from build123d import *

# Parameters (mm, degrees)
MASTER_SKETCH_R       = 52.451
MASTER_SKETCH_R_2     = 9.525
MASTER_SKETCH_R_3     = 45.974
MASTER_SKETCH_R_4     = 27.4955
MASTER_SKETCH_R_5     = 5.5
BOSS_EXTRUDE2_DEPTH   = 6.096
F_5_0MM_DOWEL_HOLE1_D = 5
CIRPATTERN4_COUNT     = 4
M6_CLEARANCE_HOLE4_D  = 6.6
M8_CLEARANCE_HOLE1_D  = 9
CIRPATTERN3_COUNT     = 18
CUT_EXTRUDE1_DEPTH    = 284.854467488


with BuildPart() as part:
    # Master Sketch → Boss-Extrude2 (new body)
    # profile 1 of 5: a face of its own
    with BuildSketch(Plane(origin=(0, 0, 0), x_dir=(1, 0, 0), z_dir=(0, 1, 0))):
        with BuildLine():
            ThreePointArc((-8.636, 127), (-36.396097826, 84.787887478), (-86.152093601, 93.552952189))
            Line((-86.152093601, 93.552952189), (-6.534964144, 18.470363023))
            ThreePointArc((-6.534964144, 18.470363023), (-3.773598517, 34.145603423), (9.525, 25.4))
            ThreePointArc((9.525, 25.4), (8.799952547, 21.754940307), (6.735192091, 18.664807909))
            Line((6.735192091, 18.664807909), (34.255961574, 46.185577392))
            ThreePointArc((34.255961574, 46.185577392), (59.945142207, 60.02346539), (89.010077776, 57.44457682))
            Line((89.010077776, 57.44457682), (207.987004211, 9.951947906))
            ThreePointArc((207.987004211, 9.951947906), (204.851852042, 25.601533276), (220.43444462, 22.148779315))
            Line((220.43444462, 22.148779315), (189.133864847, 105.44289655))
            ThreePointArc((189.133864847, 105.44289655), (188.207777178, 115.4635324), (192.51641215, 124.557840832))
            Line((192.51641215, 124.557840832), (212.800120602, 148.168522003))
            ThreePointArc((212.800120602, 148.168522003), (196.940842995, 150.353698677), (205.472725722, 163.899866417))
            Line((205.472725722, 163.899866417), (169.599038165, 163.514054819))
            ThreePointArc((169.599038165, 163.514054819), (163.800537316, 164.352688386), (158.531122559, 166.913779261))
            ThreePointArc((158.531122559, 166.913779261), (141.706259737, 175.147152322), (123.19, 177.9778))
            Line((123.19, 177.9778), (-54.61, 172.974))
            ThreePointArc((-54.61, 172.974), (-22.101472842, 159.508527158), (-8.636, 127))
        make_face()
        with Locations(Location((123.19, 116.0018, 0), (0, 0, 90))):
            Circle(MASTER_SKETCH_R, mode=Mode.SUBTRACT)
    # profile 2 of 5: a face of its own
    with BuildSketch(Plane(origin=(0, 0, 0), x_dir=(1, 0, 0), z_dir=(0, 1, 0))):
        with Locations((0, 25.4)):
            Circle(MASTER_SKETCH_R_2)
    # profile 3 of 5: a face of its own
    with BuildSketch(Plane(origin=(0, 0, 0), x_dir=(1, 0, 0), z_dir=(0, 1, 0))):
        with Locations((211.518208908, 18.79820239)):
            Circle(MASTER_SKETCH_R_2)
    # profile 4 of 5: a face of its own
    with BuildSketch(Plane(origin=(0, 0, 0), x_dir=(1, 0, 0), z_dir=(0, 1, 0))):
        with Locations((205.575158542, 154.375417219)):
            Circle(MASTER_SKETCH_R_2)
    # profile 5 of 5: a face of its own
    with BuildSketch(Plane(origin=(0, 0, 0), x_dir=(1, 0, 0), z_dir=(0, 1, 0))):
        with Locations((-54.61, 127)):
            Circle(MASTER_SKETCH_R_3)
        with Locations(Location((-54.61, 127, 0), (0, 0, 90))):
            Circle(MASTER_SKETCH_R_4, mode=Mode.SUBTRACT)
        with Locations(Location((-41.27121441, 90.351987789, 0), (0, 0, 90))):
            Circle(MASTER_SKETCH_R_5, mode=Mode.SUBTRACT)
        with Locations(Location((-67.94878559, 90.351987789, 0), (0, 0, 90))):
            Circle(MASTER_SKETCH_R_5, mode=Mode.SUBTRACT)
    extrude(amount=BOSS_EXTRUDE2_DEPTH)

    # Ø5.0mm Dowel Hole1 (through all)
    with Locations(Plane(origin=(0, 6.096, 0), x_dir=(1, 0, 0), z_dir=(0, 1, 0))):
        with Locations((123.19, 173.14676824)):
            f_5_0mm_dowel_hole1 = Hole(F_5_0MM_DOWEL_HOLE1_D / 2)

    # CirPattern4: Ø5.0mm Dowel Hole1 ×4 about axis
    cirpattern4_axis = Axis((123.19, 0, -116.0018), (0, 1, 0))
    for i in range(1, CIRPATTERN4_COUNT):
        add(f_5_0mm_dowel_hole1.rotate(cirpattern4_axis, i * 360 / CIRPATTERN4_COUNT), mode=Mode.SUBTRACT)

    # M6 Clearance Hole4 (through all)
    with Locations(Plane(origin=(0, 6.096, 0), x_dir=(1, 0, 0), z_dir=(0, 1, 0))):
        with Locations((205.575158542, 154.375417219), (211.518208908, 18.79820239), (0, 25.4)):
            Hole(M6_CLEARANCE_HOLE4_D / 2)

    # M8 Clearance Hole1 (through all)
    with Locations(Plane(origin=(0, 6.096, 0), x_dir=(1, 0, 0), z_dir=(0, 1, 0))):
        with Locations((-54.61, 166)):
            m8_clearance_hole1 = Hole(M8_CLEARANCE_HOLE1_D / 2)

    # CirPattern3: M8 Clearance Hole1 ×18 about axis, 10 skipped
    cirpattern3_axis = Axis((-54.61, 6.096, -127), (0, -1, 0))
    add([m8_clearance_hole1.rotate(cirpattern3_axis, i * 360 / CIRPATTERN3_COUNT) for i in range(1, CIRPATTERN3_COUNT) if i not in (1, 3, 5, 7, 8, 10, 11, 13, 15, 17)], mode=Mode.SUBTRACT)

    # Topology 1 → Cut-Extrude1 (cut, through all)
    with BuildSketch(Plane(origin=(0, 6.096, 0), x_dir=(1, 0, 0), z_dir=(0, 1, 0))):
        with BuildLine():
            ThreePointArc((67.281456447, 150.672141126), (71.26845327, 156.399210575), (75.839660388, 161.67173688))
            ThreePointArc((75.839660388, 161.67173688), (76.458883843, 165.158331399), (73.46509413, 167.049627827))
            Line((73.46509413, 167.049627827), (-14.700169403, 164.56840541))
            ThreePointArc((-14.700169403, 164.56840541), (-17.514771269, 162.678357132), (-17.018226233, 159.324596677))
            ThreePointArc((-17.018226233, 159.324596677), (-13.365554188, 154.512119056), (-10.325367902, 149.291082638))
            ThreePointArc((-10.325367902, 149.291082638), (-7.908159584, 146.693689239), (-4.474760882, 145.79863512))
            Line((-4.474760882, 145.79863512), (62.063515299, 147.671212322))
            ThreePointArc((62.063515299, 147.671212322), (65.050656221, 148.51412343), (67.281456447, 150.672141126))
        make_face()
        with BuildLine():
            ThreePointArc((68.334394598, 79.68843673), (68.764556906, 73.722595945), (63.886881332, 70.260721182))
            ThreePointArc((63.886881332, 70.260721182), (44.213471784, 64.716380715), (27.520769483, 52.920769483))
            Line((27.520769483, 52.920769483), (11.599172261, 36.999172261))
            ThreePointArc((11.599172261, 36.999172261), (9.657159805, 36.083732416), (7.576574711, 36.613457017))
            ThreePointArc((7.576574711, 36.613457017), (-0.198277171, 38.93169571), (-7.901868408, 36.386654554))
            ThreePointArc((-7.901868408, 36.386654554), (-9.966039712, 35.796197685), (-11.934040176, 36.65434491))
            Line((-11.934040176, 36.65434491), (-13.130428791, 37.782594013))
            ThreePointArc((-13.130428791, 37.782594013), (-16.07794783, 41.990645294), (-17.117143266, 47.022109982))
            Line((-17.117143266, 47.022109982), (-17.117143266, 64.392614711))
            ThreePointArc((-17.117143266, 64.392614711), (-14.042484998, 72.677709553), (-6.307254046, 76.95117678))
            Line((-6.307254046, 76.95117678), (59.587432499, 86.868574701))
            ThreePointArc((59.587432499, 86.868574701), (63.174454879, 86.315869277), (65.811602789, 83.822344916))
            ThreePointArc((65.811602789, 83.822344916), (67.034945598, 81.732168237), (68.334394598, 79.68843673))
        make_face()
        with BuildLine():
            ThreePointArc((206.458947193, 32.26142708), (204.959027962, 25.492155206), (198.160653587, 24.130206141))
            Line((198.160653587, 24.130206141), (145.349760257, 45.211000835))
            ThreePointArc((145.349760257, 45.211000835), (142.353542672, 49.714608993), (145.500239117, 54.114393959))
            ThreePointArc((145.500239117, 54.114393959), (164.91203471, 65.138555749), (179.519499105, 82.019667539))
            ThreePointArc((179.519499105, 82.019667539), (184.033435332, 84.302068881), (188.055524715, 81.234859539))
            Line((188.055524715, 81.234859539), (206.458947193, 32.26142708))
        make_face()
        with BuildLine():
            Line((190.604833072, 136.949630286), (196.435820245, 143.737027147))
            ThreePointArc((196.435820245, 143.737027147), (197.375389236, 150.556102986), (191.550890325, 154.22459009))
            Line((191.550890325, 154.22459009), (182.60327011, 154.128360907))
            ThreePointArc((182.60327011, 154.128360907), (179.873089832, 152.515317466), (179.900424771, 149.344348167))
            ThreePointArc((179.900424771, 149.344348167), (182.824339377, 143.778469401), (185.203579034, 137.958890231))
            ThreePointArc((185.203579034, 137.958890231), (187.613336253, 135.897613045), (190.604833072, 136.949630286))
        make_face()
    extrude(amount=-CUT_EXTRUDE1_DEPTH, mode=Mode.SUBTRACT)


solid = part.part
Verification items for the finished model (mm, model axes). A direction names the side the tool comes from. Coordinates: 2 decimals unless noted, no trailing zeros. Write each loop counter-clockwise with the first axis right and the second up, starting at its lowest first coordinate (ties: lowest second). Pieces come first, ordered by that corner, then holes. Notation, with made-up numbers: (41, 84.25) -> (53, 84.25) arc R9 ccw to (53, 101.25) -> close; hole circle Ø11 at (15.5, 12.5). An arc over 180 degrees is marked (long way). One line per item, written item: value. Start each with the question number.
Q1. Thickness scan on L1, parallel to Z at x = 6.5, y = 5.25; L2, parallel to X at y = 6, z = -113; L3, parallel to X at y = 4, z = -125. Record the ranges inside material, lowest first. Write a range as from..to.
Q2. Cross-section at C-C on y = 5. State how many separate pieces and enclosed holes the cut face has, and give its area (3 significant figures).
Q3. Mould release check, pull along X, two halves, no side actions. Record for faces 1 (the cylindrical face through (-97.05, 3.01, -144.68)), 2 (the cylindrical face through (-13.41, 3.09, -154.58)), 3 (the cylindrical face through (218.074, 3.005, -11.888)): pulls with the +X half, pulls with the -X half, needs draft (parallel to the pull), parting line crosses it, or undercut.
Q4. Access from +Z, -Z, +X, -X, +Y, -Y to the whole of each face (thin tool, end or side, straight path). Record for faces 4 (the cylindrical face through (71.208, 3.091, -156.322)), 5 (the cylindrical face through (163.88, 3.01, -164.33)), 6 (the flat face through (147.67, 3.01, -34.03)).
Q5. Cross-section at B-B on x = 111.5. Enter the section's corners in (y, z), and give its area (3 significant figures).
Q6. Go/stop test with flat-tipped pins: P1, Ø9, axis at x = -41.27, z = -90.35, coming from the +Y side; P2, Ø3, axis at y = 3, z = -53.5, coming from the +X side; P3, Ø2, axis at x = 176.5, y = 3, coming from the +Z side; P4, Ø3, axis at y = 3, z = -59, coming from the +X side. Record where each tip stops, or that it passes through.
Q7. Cross-section at A-A on x = 0. Enter the section's corners in (y, z) (3 decimals), and give its area (3 significant figures).
Checked values:
1. L1: z = -174.69..-165.17, -146.11..-78.88, -37.27..-18.44
1. L2: x = -98.4..-78.27, -30.95..70.82, 175.56..187.94
1. L3: x = -100.54..-82.03, -27.19..71.52, 174.86..192.9
2. separate pieces: 1
2. enclosed holes: 23
2. area: 20,000 mm²
3. face 1: pulls with the -X half
3. face 2: undercut
3. face 3: parting line crosses it
4. face 4: +Y, -Y
4. face 5: -Z, +Y, -Y
4. face 6: +Z, +Y, -Y
5. outline: (0, -177.65) -> (6.1, -177.65) -> (6.1, -167.13) -> (0, -167.13) -> close; (0, -64.87) -> (6.1, -64.87) -> (6.1, -48.47) -> (0, -48.47) -> close
5. area: 164 mm²
6. P1: passes through
6. P2: stops at x = 209.22
6. P3: stops at z = -22.12
6. P4: stops at x = 207.15
7. outline: (0, -174.511) -> (6.096, -174.511) -> (6.096, -164.982) -> (0, -164.982) -> close; (0, -145.925) -> (6.096, -145.925) -> (6.096, -77.9) -> (0, -77.9) -> close; (0, -38.933) -> (6.096, -38.933) -> (6.096, -28.7) -> (0, -28.7) -> close; (0, -22.1) -> (6.096, -22.1) -> (6.096, -15.875) -> (0, -15.875) -> close
7. area: 573 mm²
